```python
from build123d import *

# Parameters (mm, degrees)
CROQUIS1_R                 = 13
CROQUIS1_R_2               = 9.35
SALIENTE_EXTRUIR1_DEPTH    = 40
CROQUIS1_2_R               = 13
CROQUIS1_2_R_2             = 9.35
SALIENTE_EXTRUIR2_DEPTH    = 16
CROQUIS2_R                 = 6.5
SALIENTE_EXTRUIR3_DEPTH    = 22
REDONDEO1_R                = 0.5
REDONDEO2_R                = 0.5
CROQUIS3_R                 = 2.75
CORTAR_EXTRUIR1_DEPTH      = 45.022721406
CORTAR_EXTRUIR1_DEPTH_BACK = 45.022721406


with BuildPart() as part:
    # Croquis1 → Saliente-Extruir1 (new body)
    with BuildSketch(Plane.XY):
        Circle(CROQUIS1_R)
        Circle(CROQUIS1_R_2, mode=Mode.SUBTRACT)
    extrude(amount=SALIENTE_EXTRUIR1_DEPTH)

    # Croquis1_2 → Saliente-Extruir2 (add)
    with BuildSketch(Plane.XY):
        Circle(CROQUIS1_2_R)
        Circle(CROQUIS1_2_R_2, mode=Mode.SUBTRACT)
        Circle(CROQUIS1_2_R_2)
    extrude(amount=-SALIENTE_EXTRUIR2_DEPTH)

    # Croquis2 → Saliente-Extruir3 (add)
    with BuildSketch(Plane(origin=(0, 0, -16), x_dir=(-1, 0, 0), z_dir=(0, 0, -1))):
        Circle(CROQUIS2_R)
    extrude(amount=SALIENTE_EXTRUIR3_DEPTH)

    # Redondeo1
    redondeo1_edges = [part.edges().sort_by_distance(p)[0] for p in [
        (6.5, 0, -16),
    ]]
    fillet(redondeo1_edges, radius=REDONDEO1_R)

    # Redondeo2
    redondeo2_edges = [part.edges().sort_by_distance(p)[0] for p in [
        (-9.35, 0, 0),
    ]]
    fillet(redondeo2_edges, radius=REDONDEO2_R)

    # Croquis3 → Cortar-Extruir1 (cut, two sides)
    with BuildSketch(Plane(origin=(0, 0, 0), x_dir=(1, 0, 0), z_dir=(0, 1, 0))) as cortar_extruir1_sk:
        with Locations(Location((0, 9.25, 0), (0, 0, 270))):
            Circle(CROQUIS3_R)
    extrude(amount=CORTAR_EXTRUIR1_DEPTH, mode=Mode.SUBTRACT)
    extrude(cortar_extruir1_sk.sketch, amount=-CORTAR_EXTRUIR1_DEPTH_BACK, mode=Mode.SUBTRACT)


solid = part.part
```
Geometry check sheet. Reference: the model listing, model coordinates, mm. A direction names the side the tool comes from. Round coordinates to 2 decimals unless told otherwise and drop trailing zeros. Loops run counter-clockwise (first coordinate to the right, second up) from the corner with the lowest first, then second, coordinate; pieces in that order, holes last. Notation, with made-up numbers: (61, 1) -> (116, 1) arc R19 cw to (116, 18) -> close; hole circle Ø10 at (-26, 87.25). An arc over 180 degrees is marked (long way). Use a Markdown table: item, result.
(1) Mould release check, pull along X, two halves, no side actions. Record for faces 1 (the flat face through (6, -8, 40)), 2 (the flat face through (0, 0, 0)), 3 (the cylindrical face through (5.158, -3.955, -27.1)): released by +X, released by -X, zero draft, split by the parting line, or undercut.
Calculated:
| item | result |
|---|---|
| face 1 | zero draft |
| face 2 | undercut |
| face 3 | split by the parting line |
(2) Sectioned sample at C-C (z = -24). Enter the section's corners in (x, y), then the cut area to 3 significant figures.
Calculated:
| item | result |
|---|---|
| outline | circle Ø13 at (0, 0) |
| area | 133 mm² |
(3) Sectioned sample at A-A (x = 0). Enter the section's corners in (y, z).
Calculated:
| item | result |
|---|---|
| outline | (-13, -16) -> (-7, -16) arc R0.5 cw to (-6.5, -16.5) -> (-6.5, -38) -> (6.5, -38) -> (6.5, -16.5) arc R0.5 cw to (7, -16) -> (13, -16) -> (13, -12) -> (-13, -12) -> close; (-13, -6.5) -> (13, -6.5) -> (13, 40) -> (9.35, 40) -> (9.35, 0.5) arc R0.5 cw to (8.85, 0) -> (-8.85, 0) arc R0.5 cw to (-9.35, 0.5) -> (-9.35, 40) -> (-13, 40) -> close |
(4) Go/stop test with flat-tipped pins: P1, Ø6, axis at x = 10, z = -15, coming from the +Y side; P2, Ø1.5, axis at x = -10, y = -3, coming from the -Z side; P3, Ø1.5, axis at x = -6.5, z = -0.5, coming from the -Y side. Record where each tip stops, or that it passes through.
Calculated:
| item | result |
|---|---|
| P1 | y = 10.95 |
| P2 | z = -16 |
| P3 | y = -11.66 |
(5) Sectioned sample at B-B (y = 0). Enter the section's corners in (x, z), then the cut area to 3 significant figures.
Calculated:
| item | result |
|---|---|
| outline | (-13, -16) -> (-7, -16) arc R0.5 cw to (-6.5, -16.5) -> (-6.5, -38) -> (6.5, -38) -> (6.5, -16.5) arc R0.5 cw to (7, -16) -> (13, -16) -> (13, 40) -> (9.35, 40) -> (9.35, 0.5) arc R0.5 cw to (8.85, 0) -> (-8.85, 0) arc R0.5 cw to (-9.35, 0.5) -> (-9.35, 40) -> (-13, 40) -> close; hole circle Ø5.5 at (0, -9.25) |
| area | 970 mm² |
(6) Scan lines: probe 1 along Y at (x, z) = (0, 17); probe 2 along Z at (x, y) = (0, 0.25); probe 3 along X at (y, z) = (-1, 36). Record each from-to range of solid material in increasing order.
Calculated:
| item | result |
|---|---|
| probe 1 | -13 to -9.35, 9.35 to 13 |
| probe 2 | -38 to -12, -6.5 to 0 |
| probe 3 | -12.96 to -9.3, 9.3 to 12.96 |
(7) Set-up check for faces 4 (the flat face through (6, -6, -16)), 5 (the cylindrical face through (-1.05, 0.18, -6.71)), 6 (the cylindrical face through (-2.027, -9.128, 19.974)): record each of +Z, -Z, +X, -X, +Y, -Y from which the full face is reachable in a straight line by a thin tool's end or side.
Calculated:
| item | result |
|---|---|
| face 4 | -Z |
| face 5 | +Y, -Y |
| face 6 | +Z |
(8) Sectioned sample at D-D (y = 11.5). Enter the section's corners in (x, z), then the cut area to 3 significant figures.
Calculated:
| item | result |
|---|---|
| outline | (-6.06, -16) -> (6.06, -16) -> (6.06, 40) -> (-6.06, 40) -> close; hole circle Ø5.5 at (0, -9.25) |
| area | 655 mm² |
